```python
from build123d import *

# Parameters (mm, degrees)
BOSS_EXTRUDE1_DEPTH = 6
BOSS_EXTRUDE2_DEPTH = 20
SKETCH4_RX          = 4.5
SKETCH4_RY          = 4
CUT_EXTRUDE1_DEPTH  = 15
SKETCH5_R           = 11
CUT_EXTRUDE2_DEPTH  = 30
BOSS_EXTRUDE3_DEPTH = 13


with BuildPart() as part:
    # Sketch1 → Revolve1 (revolve)
    with BuildSketch(Plane.XY):
        Polygon((0, 0), (162, 0), (162, 12.5), (58, 14.5), (58, 9), (25, 9), (25, 6.5), (15, 6.5), (15, 5.5), (0, 5.5), align=None)
    revolve(axis=Axis((0, 0, 0), (1, 0, 0)))

    # Sketch2 → Boss-Extrude1 (add)
    with BuildSketch(Plane.ZY.offset(-15)):
        Polygon((0, 8.082903769), (-7, 4.041451884), (-7, -4.041451884), (0, -8.082903769), (7, -4.041451884), (7, 4.041451884), align=None)
    extrude(amount=-BOSS_EXTRUDE1_DEPTH)

    # Sketch3 → Boss-Extrude2 (add)
    with BuildSketch(Plane.ZY.offset(-58)):
        Polygon((5.773502692, 10), (-5.773502692, 10), (-11.547005384, 0), (-5.773502692, -10), (5.773502692, -10), (11.547005384, 0), align=None)
    extrude(amount=BOSS_EXTRUDE2_DEPTH)

    # Sketch4 → Cut-Extrude1 (cut, symmetric)
    with BuildSketch(Plane(origin=(0, 0, 0), x_dir=(1, 0, 0), z_dir=(0, 1, 0))):
        with Locations(Location((162, 0), (0, 0, 90))):
            Ellipse(SKETCH4_RX, SKETCH4_RY)
    extrude(amount=CUT_EXTRUDE1_DEPTH, both=True, mode=Mode.SUBTRACT)

    # Sketch5 → Cut-Extrude2 (cut)
    with BuildSketch(Plane(origin=(162, 0, 0), x_dir=(0, 0, -1), z_dir=(1, 0, 0))):
        Circle(SKETCH5_R)
    extrude(amount=-CUT_EXTRUDE2_DEPTH, mode=Mode.SUBTRACT)

    # Sketch6 → Boss-Extrude3 (add)
    with BuildSketch(Plane.XZ.offset(-10)):
        Polygon((48, 7.505553499), (41.5, 3.75277675), (41.5, -3.75277675), (48, -7.505553499), (54.5, -3.75277675), (54.5, 3.75277675), align=None)
    boss_extrude3 = extrude(amount=-BOSS_EXTRUDE3_DEPTH)

    # Mirror1: Boss-Extrude3 across plane
    add(boss_extrude3.mirror(Plane.ZX))


solid = part.part
```
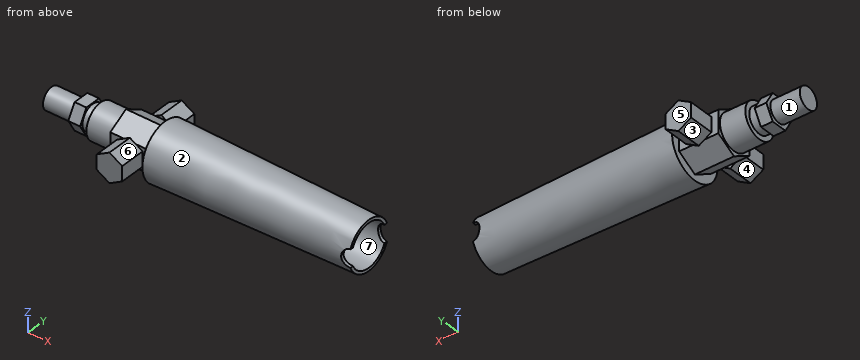
For this review, take the finished solid that the model builds, in its own axes (mm). Face numbers are marked on the shaded views. A direction names the side the tool comes from. Round coordinates to 2 decimals unless told otherwise and drop trailing zeros. Loops run counter-clockwise (first coordinate to the right, second up) from the corner with the lowest first, then second, coordinate; pieces in that order, holes last.
Q1. Add section C-C on x = 28. Write out the cut boundary in (y, z), plus the area to 3 significant figures.
Result sheet:
outline: circle Ø18 at (0, 0)
area: 254 mm2
Q2. Add section A-A on x = 141. Write out the cut boundary in (y, z), plus the area to 3 significant figures.
Result sheet:
outline: circle Ø25.81 at (0, 0); hole circle Ø22 at (0, 0)
area: 143 mm2
Q3. Machinability: for the marked faces 1, 2, 3 and 4, which of the approach directions +Z, -Z, +X, -X, +Y, -Y give a long, thin tool a straight path to every point of the face, cutting with its end or side? Answer none if there is none.
Result sheet:
face 1: -X
face 2: +X
face 3: -Z, -X, +Y
face 4: -Z, -X, -Y
Q4. Insertion check: pin 1 Ø4 at (y, z) = (-15, 0.5) entering from -X; pin 2 Ø10 at (y, z) = (13, 8.5) entering from -X; pin 3 Ø1.5 at (x, z) = (124, -4) entering from -Y. Each pin has a flat end and moves straight along its axis. Give the tip position at first contact, or say it passes through.
Result sheet:
pin 1: stops at x = 41.5
pin 2: stops at x = 38
pin 3: stops at y = -12.83
Q5. Mouldability with a two-part tool opening along Y and no side actions: class the marked faces 5, 6 and 7 as +Y half, -Y half, draft (parallel to the pull), parting line (faces both ways), or undercut.
Result sheet:
face 5: +Y half
face 6: draft
face 7: undercut
Q6. Add section B-B on x = 110. Write out the cut boundary in (y, z), plus the area to 3 significant figures.
Result sheet:
outline: circle Ø27 at (0, 0)
area: 573 mm2
Q7. To check wall thickness, follow line 1 along X through (y, z) = (-8.5, -5.5); line 2 along X through (y, z) = (-0.5, -0.5); line 3 along Z through (x, y) = (153, 0). State the ranges of each line that lie inside material, in increasing order.
Result sheet:
line 1: x = 38 to 132
line 2: x = 0 to 132
line 3: z = -12.67 to -11, 11 to 12.67
